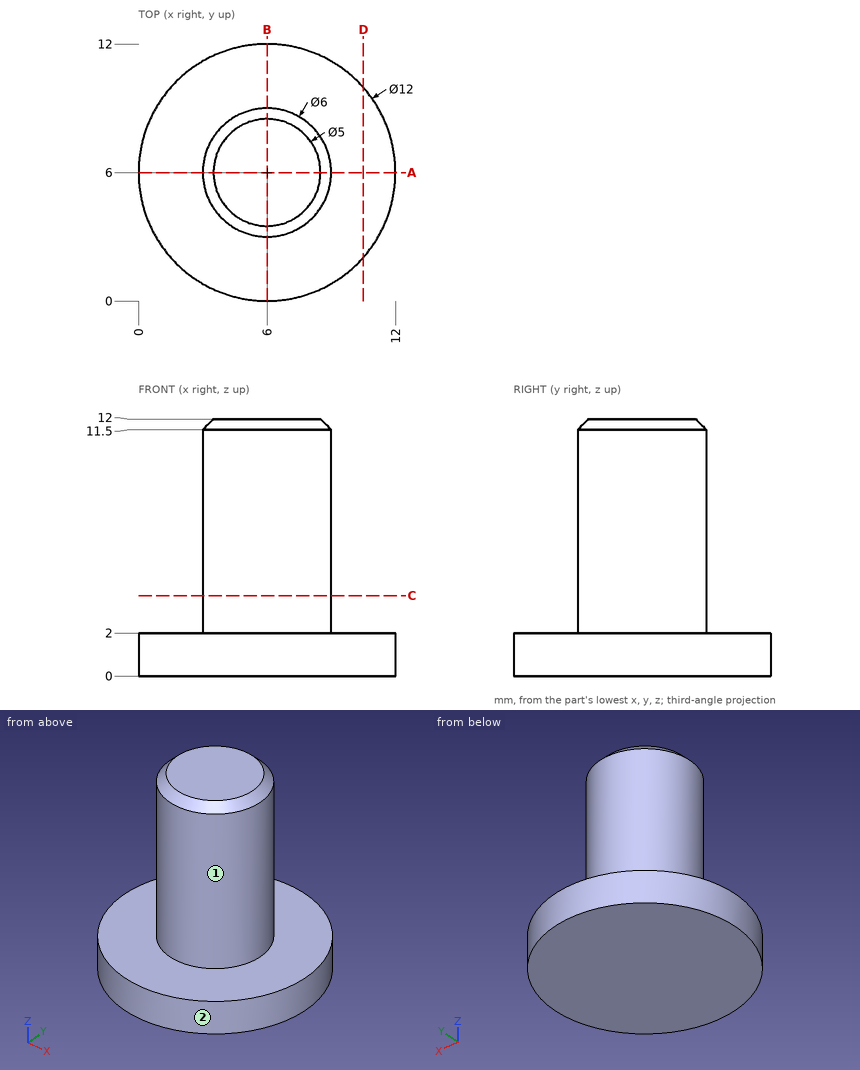
Geometry: see drawing. Coordinates: mm, zero at the bounding-box minimum. A direction names the side the tool comes from. Round coordinates to 2 decimals unless told otherwise and drop trailing zeros. Order: outer loops, then holes, each group sorted by start corner. A loop starts at its lowest first (then second) coordinate and runs counter-clockwise, first axis right, second up. Notation, with made-up numbers: (1, 86) - (17, 86) arc R13 ccw to (17, 109) - close; hole circle Ø10 at (54.25, 22.5). An arc over 180 degrees is marked (long way). Use a Markdown table: item, result. Add a question column.
1. First-contact query: pin 1 (6 mm diameter, centred on y = 10, z = 7.5, fed in from -X); pin 2 (2 mm diameter, centred on y = 5.5, z = 10.5, fed in from +X); pin 3 (5 mm diameter, centred on y = 1.5, z = 7, fed in from +X). Flat tips, straight axial feed; report the tip coordinate or a pass-through.
2. Section query A-A (y = 6). Return the cut outline in (x, z).
3. Line query: probe 1 along Z at (x, y) = (11.25, 3.75); probe 2 along X at (y, z) = (4, 3.25); probe 3 along X at (y, z) = (7.75, 1.25). Output: solid intervals per line, ascending.
4. Section query C-C (z = 3.75). Return the cut outline in (x, y).
5. Section query D-D (x = 10.5). Return the cut outline in (y, z).
6. Set-up query: the marked faces 1 and 2. Return all of +Z, -Z, +X, -X, +Y, -Y with unobstructed straight access to the full face (end or side cutting, diameter ignored); none if empty.
Derived:
| question | item | result |
|---|---|---|
| 1 | pin 1 | x = 3.17 |
| 1 | pin 2 | x = 9 |
| 1 | pin 3 | x = 8.24 |
| 2 | outline | (0, 0) - (12, 0) - (12, 2) - (9, 2) - (9, 11.5) - (8.5, 12) - (3.5, 12) - (3, 11.5) - (3, 2) - (0, 2) - close |
| 3 | probe 1 | 0 to 2 |
| 3 | probe 2 | 3.76 to 8.24 |
| 3 | probe 3 | 0.26 to 11.74 |
| 4 | outline | circle Ø6 at (6, 6) |
| 5 | outline | (2.03, 0) - (9.97, 0) - (9.97, 2) - (2.03, 2) - close |
| 6 | face 1 | +Z |
| 6 | face 2 | +Z, -Z |
